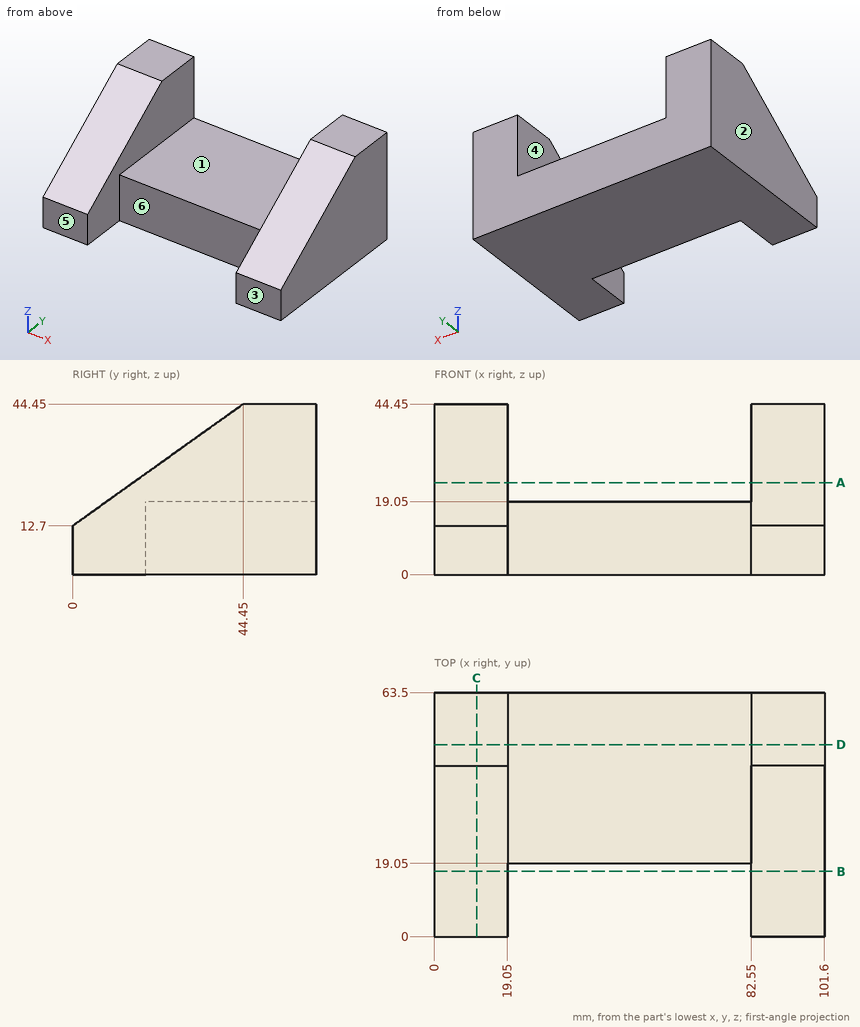
Job drawing, mm, ordinate dimensions from the low corner. One solid piece. A direction names the side the tool comes from. Give positions to 0.01 mm unless a question says otherwise; leave off trailing zeros. Order: outer loops, then holes, each group sorted by start corner. A loop starts at its lowest first (then second) coordinate and runs counter-clockwise, first axis right, second up. Notation, with made-up numbers: M 75,5.5 L 92,5.5 A23 ccw 92,44.5 Z; hole C 76.5,71 d6. An arc over 180 degrees is marked long. Return JSON: item names as keys, results as strings.
Q1. Flat gauge pins, fed straight in: pin 1 (9.5 mm diameter, centred on x = 47, z = 13.5, fed in from -Y); pin 2 (8 mm diameter, centred on y = 36, z = 10, fed in from -X); pin 3 (12 mm diameter, centred on x = 71.5, y = 28.5, fed in from +Z). Where does each tip first touch, or does it go through?
Answer list:
{"pin 1": "stops at y = 19.05", "pin 2": "stops at x = 0", "pin 3": "stops at z = 19.05"}
Q2. Band-saw the part on A-A (z = 24). Give the cut face in (x, y), then the cut area to 3 significant figures.
Answer list:
{"outline": "M 0,15.82 L 19.05,15.82 L 19.05,63.5 L 0,63.5 Z; M 82.55,15.82 L 101.6,15.82 L 101.6,63.5 L 82.55,63.5 Z", "area": "1,820 mm^2"}
Q3. Band-saw the part on B-B (y = 17). Give the cut face in (x, z).
Answer list:
{"outline": "M 0,0 L 19.05,0 L 19.05,24.84 L 0,24.84 Z; M 82.55,0 L 101.6,0 L 101.6,24.84 L 82.55,24.84 Z"}
Q4. 3-axis set-ups, long thin cutter, end or side, ignore diameter. For the marked faces 4, 5 and 6: which of +Z, -Z, +X, -X, +Y, -Y reach the whole face in a straight line?
Answer list:
{"face 4": "+Z, -Y", "face 5": "+Z, -Z, +X, -X, -Y", "face 6": "+Z, -Z, -Y"}
Q5. Band-saw the part on C-C (x = 11). Give the cut face in (y, z).
Answer list:
{"outline": "M 0,0 L 63.5,0 L 63.5,44.45 L 44.45,44.45 L 0,12.7 Z"}
Q6. Two-plate mould, pull along X, no slides. Class the marked faces 1, 2 and 3: pulls with the +X half, pulls with the -X half, needs draft (parallel to the pull), parting line crosses it, or undercut.
Answer list:
{"face 1": "undercut", "face 2": "pulls with the -X half", "face 3": "needs draft"}
Q7. Band-saw the part on D-D (y = 50). Give the cut face in (x, z).
Answer list:
{"outline": "M 0,0 L 101.6,0 L 101.6,44.45 L 82.55,44.45 L 82.55,19.05 L 19.05,19.05 L 19.05,44.45 L 0,44.45 Z"}
Q8. Wall check: probe 1 along X at (y, z) = (37, 26.5); probe 2 along Y at (x, z) = (23.5, 11); probe 3 along Z at (x, y) = (53, 52.5). Give the ranges that are in metal, low to high. Write a range as from..to.
Answer list:
{"probe 1": "x = 0..19.05, 82.55..101.6", "probe 2": "y = 19.05..63.5", "probe 3": "z = 0..19.05"}
